CAD build for the part. Positions are in the model's coordinates, mm. Face numbers are marked on the shaded views. A direction names the side the tool comes from. Round coordinates to 2 decimals unless told otherwise and drop trailing zeros. Order: outer loops, then holes, each group sorted by start corner. A loop starts at its lowest first (then second) coordinate and runs counter-clockwise, first axis right, second up. Notation, with made-up numbers: M 55,82.5 L 80,82.5 A22 cw 80,119.5 Z; hole C 35,70.5 d9. An arc over 180 degrees is marked long. Answer as a JSON object with one key per item and string values.
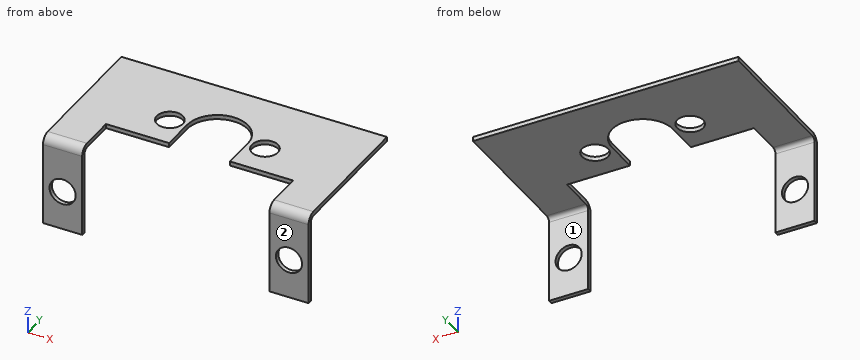
```python
from build123d import *

# Parameters (mm, degrees)
BRIDA_BASE1_DEPTH     = 30.5
CROQUIS12_R           = 1.5
CORTAR_EXTRUIR1_DEPTH = 12
CROQUIS13_R           = 1.5
CORTAR_EXTRUIR2_DEPTH = 12


# Sheet-metal steps are written as plain solids
with BuildPart() as part:
    # Croquis1 → Brida base1 (new body)
    with BuildSketch(Plane(origin=(0, 0, 0), x_dir=(0, 0, -1), z_dir=(1, 0, 0))):
        with BuildLine():
            Line((-59.724940778, -1.485262267), (-59.724940778, -16.985262267))
            ThreePointArc((-59.724940778, -16.985262267), (-59.578494169, -17.338815658), (-59.224940778, -17.485262267))
            Line((-59.224940778, -17.485262267), (-49.724940778, -17.485262267))
            Line((-49.724940778, -17.485262267), (-49.724940778, -17.985262267))
            Line((-49.724940778, -17.985262267), (-59.224940778, -17.985262267))
            ThreePointArc((-59.224940778, -17.985262267), (-59.93204756, -17.692369049), (-60.224940778, -16.985262267))
            Line((-60.224940778, -16.985262267), (-60.224940778, -1.485262267))
            Line((-60.224940778, -1.485262267), (-59.724940778, -1.485262267))
        make_face()
    extrude(amount=BRIDA_BASE1_DEPTH)

    # Croquis12 → Cortar-Extruir1 (cut)
    with BuildSketch(Plane.XY.offset(60.224940778)):
        with Locations((9.79, -9.235262267)):
            Circle(CROQUIS12_R)
        with Locations(Location((20.71, -9.235262267, 0), (0, 0, 90))):
            Circle(CROQUIS12_R)
        with BuildLine():
            Line((11.75, -9.235262267), (11.75, -12.985262267))
            Line((11.75, -12.985262267), (4.5, -12.985262267))
            Line((4.5, -12.985262267), (4.5, -17.985262267))
            Line((4.5, -17.985262267), (11.75, -17.985262267))
            Line((11.75, -17.985262267), (18.75, -17.985262267))
            Line((18.75, -17.985262267), (26, -17.985262267))
            Line((26, -17.985262267), (26, -12.985262267))
            Line((26, -12.985262267), (18.75, -12.985262267))
            Line((18.75, -12.985262267), (18.75, -9.235262267))
            ThreePointArc((18.75, -9.235262267), (15.25, -5.735262267), (11.75, -9.235262267))
        make_face()
    extrude(amount=-CORTAR_EXTRUIR1_DEPTH, mode=Mode.SUBTRACT)

    # Croquis13 → Cortar-Extruir2 (cut)
    with BuildSketch(Plane(origin=(0, -17.485262267, 0), x_dir=(-1, 0, 0), z_dir=(0, 1, 0))):
        with Locations(Location((-28.25, 54.224940778, 0), (0, 0, 90))):
            Circle(CROQUIS13_R)
        with Locations(Location((-2.25, 54.224940778, 0), (0, 0, 90))):
            Circle(CROQUIS13_R)
    extrude(amount=-CORTAR_EXTRUIR2_DEPTH, mode=Mode.SUBTRACT)


solid = part.part
```
Item 1: Saw through at A-A on x = 20.71. List the corners of the cut face in (y, z).
Worked answers:
{"outline": "M -12.99,59.72 L -10.74,59.72 L -10.74,60.22 L -12.99,60.22 Z; M -7.74,59.72 L -1.49,59.72 L -1.49,60.22 L -7.74,60.22 Z"}
Item 2: Wall check: line 1 along Y through (x, z) = (9.79, 60.05); line 2 along Y through (x, z) = (26.5, 53.75); line 3 along Z through (x, y) = (23, -7.5). Give the ranges that are in metal, low to high. Write a range as [from, to].
Worked answers:
{"line 1": "y = [-12.99, -10.74], [-7.74, -1.49]", "line 2": "y = [-17.99, -17.49]", "line 3": "z = [59.72, 60.22]"}
Item 3: Drop flat-ended pins along their axis: pin 1 Ø1.3 at (x, z) = (27.5, 55.5) entering from +Y; pin 2 Ø4.5 at (x, y) = (16, -5.5) entering from -Z; pin 3 Ø6 at (x, z) = (21, 57) entering from +Y. Give the stop position or say it passes through.
Worked answers:
{"pin 1": "stops at y = -17.49", "pin 2": "stops at z = 59.72", "pin 3": "stops at y = -1.49"}
Item 4: Saw through at D-D on x = 28.25. List the corners of the cut face in (y, z).
Worked answers:
{"outline": "M -17.99,49.72 L -17.49,49.72 L -17.49,52.72 L -17.99,52.72 Z; M -17.99,55.72 L -17.49,55.72 L -17.49,59.22 A0.5 cw -16.99,59.72 L -1.49,59.72 L -1.49,60.22 L -16.99,60.22 A1 ccw -17.99,59.22 Z"}
Item 5: Saw through at B-B on z = 58.5. List the corners of the cut face in (x, y).
Worked answers:
{"outline": "M 0,-17.99 L 4.5,-17.99 L 4.5,-17.49 L 0,-17.49 Z; M 26,-17.99 L 30.5,-17.99 L 30.5,-17.49 L 26,-17.49 Z"}
Item 6: 3-axis set-ups, long thin cutter, end or side, ignore diameter. For the marked faces 1 and 2: which of +Z, -Z, +X, -X, +Y, -Y reach the whole face in a straight line?
Worked answers:
{"face 1": "-Z, +X, -X, +Y", "face 2": "+Z, -Z, +X, -X, -Y"}
Item 7: Saw through at C-C on y = -10. List the corners of the cut face in (x, z).
Worked answers:
{"outline": "M 0,59.72 L 8.5,59.72 L 8.5,60.22 L 0,60.22 Z; M 11.08,59.72 L 11.75,59.72 L 11.75,60.22 L 11.08,60.22 Z; M 18.75,59.72 L 19.42,59.72 L 19.42,60.22 L 18.75,60.22 Z; M 22,59.72 L 30.5,59.72 L 30.5,60.22 L 22,60.22 Z"}
